Autodesk Inventor part; units mm, degrees
ref_plane "WorkPlane1" through (0, 0, 0) normal (0, 0, 1) x (1, 0, 0)
ref_plane "MSC_PF1" through (0, 0, 0) normal (1, 0, 0) x (0, 1, 0)
ref_plane "MSC_PT1" through (0, 0, 0) normal (0, 0, -1) x (-1, 0, 0)
ref_plane "WorkPlane1" through (0, 0, 0) normal (0, 0, 1) x (1, 0, 0)
sketch "Szkic1" plane through (0, 0, 0) normal (0, 0, 1) x (1, 0, 0)
  point P0 (0, 0)
sketch "Szkic2" plane through (0, 0, 0) normal (0, 0, 1) x (1, 0, 0)
  line L0 (-6.5, 3.7529) -> (-6.5, -3.7529)
  line L1 (0, 7.5054) -> (-6.5, 3.7529)
  line L2 (6.5, 3.7529) -> (0, 7.5054)
  line L3 (6.5, -3.7529) -> (6.5, 3.7529)
  line L4 (0, -7.5054) -> (6.5, -3.7529)
  line L5 (-6.5, -3.7529) -> (0, -7.5054)
  circle A0 centre (0, 0) radius 6.5 construction
  dimension "d1" = 13
  dimension "d29" = 0
  dimension "d30" = 0
extrude "Wyciągnięcie proste1" add sketch "Szkic2" along normal blind 5.3
sketch "Szkic3" plane through (0, 0, 0) normal (1, 0, 0) x (0, 1, 0)
  line L0 (6.5, 5.3) -> (7.6054, 5.3)
  line L1 (7.6054, 4.6618) -> (6.5, 5.3)
  line L2 (7.6054, 5.3) -> (7.6054, 4.6618)
  line L3 (0, -1.06) -> (0, 6.36)
  line L4 (7.5054, 0) -> (7.5054, 5.3)
  dimension "d25" = 0.1
  dimension "d26" = 0
  dimension "d27" = 60
  dimension "d28" = 6.5
revolve "Obrót1" cut sketch "Szkic3" angle 360 about axis through (0, 0, -10) along (0, 0, 1)
sketch "Szkic4" plane through (0, 0, 0) normal (1, 0, 0) x (0, 1, 0)
  line L0 (0, -65) -> (0, 0)
  line L1 (-4, -65) -> (0, -65)
  line L2 (-4, 0) -> (-4, -65)
  line L3 (0, 0) -> (-4, 0)
  line L4 (0, -65) -> (0, 0)
  line L5 (-4.8, 0) -> (0.8, 0)
  line L6 (0, -78) -> (0, 13)
  dimension "d18" = 4
  dimension "d20" = 65
  dimension "d33" = 0
  dimension "d34" = 0
revolve "Obrót2" add sketch "Szkic4" angle 360 about axis through (0, 0, -65) along (0, 0, -1)
chamfer "Faza1" distance 0.625 angle 45 1 edges at (0, 4, -65)
fillet "Zaokrąglenie1" radius 0.4 1 edges at (0, 4, 0)
thread "Gwint1"
ref_plane "MSC_PF1" through (0, 0, 0) normal (1, 0, 0) x (0, 1, 0)
ref_plane "MSC_PT1" through (0, 0, 0) normal (0, 0, -1) x (-1, 0, 0)
equation "\"d1\" = ParS"
equation "\"d6\" = ParK"
equation "\"d22\" = 0.5 * PTC"
equation "\"d23\" = 0.5 * PTC"
equation "\"d24\" = r"
equation "\"d28\" = 0.5 * ParS"
equation "\"d18\" = 0.5 * NND"
equation "\"d20\" = NLG"
equation "\"NND\" = 8"
equation "\"NLG\" = 65"
equation "\"PTC\" = 1.25"
equation "\"ParK\" = 5.3"
equation "\"ParS\" = 13"
equation "\"msp_es\" = 0.577367 * ParS"
equation "\"r\" = 0.4"
equation "\"THREADDIA\" = NND"
properties part number "ISO 4016 - M8 x 65" material "Stal"
Geometry check sheet. Reference: the model listing, model coordinates, mm. A direction names the side the tool comes from. Round coordinates to 2 decimals unless told otherwise and drop trailing zeros. Order: outer loops, then holes, each group sorted by start corner. A loop starts at its lowest first (then second) coordinate and runs counter-clockwise, first axis right, second up. Notation, with made-up numbers: (7, 25.25) - (23, 25.25) arc R15 cw to (23, 35.25) - close; hole circle Ø10 at (18.25, 69.25). An arc over 180 degrees is marked (long way). Use a Markdown table: item, result. Add a question column.
(1) Depth check by flat-ended pin: pin 1 (1 mm diameter, centred on x = -3.5, y = 5, fed in from -Z); pin 2 (1 mm diameter, centred on x = -4, z = -36, fed in from +Y); pin 3 (6 mm diameter, centred on x = 0.5, z = -42.5, fed in from +Y). Enter the tip coordinate at first touch or a pass-through.
(2) Sectioned sample at A-A, the plane z = -14.5. Enter the section's corners in (x, y).
(3) Tool access check on faces 1 (the flat face through (-6.5, 0, 3)), 2 (the cylindrical face through (3.905, 0.867, -32.835)). Record the directions out of +Z, -Z, +X, -X, +Y, -Y that give a thin tool (end or side, any length) a straight path to the whole face; none if there is none.
(4) Material ranges on line 1 along Z through (x, y) = (-4.5, -0.75); line 2 along X through (y, z) = (0.25, -33); line 3 along Y through (x, z) = (-0.5, -25), recorded low to high. Write a range as [from, to].
Answers below:
| question | item | result |
|---|---|---|
| 1 | pin 1 | z = 0 |
| 1 | pin 2 | y = 1.94 |
| 1 | pin 3 | y = 4 |
| 2 | outline | circle Ø8 at (0, 0) |
| 3 | face 1 | +Z, -Z, -X, +Y, -Y |
| 3 | face 2 | -Z |
| 4 | line 1 | [0, 5.3] |
| 4 | line 2 | [-3.99, 3.99] |
| 4 | line 3 | [-3.97, 3.97] |
